```python
from build123d import *

# Parameters (mm, degrees)
SKETCH4_R           = 63.754
BOSS_EXTRUDE1_DEPTH = 62.5856
SKETCH5_R           = 34.671
BOSS_EXTRUDE2_DEPTH = 58.42


with BuildPart() as part:
    # Sketch1 → Revolve1 (revolve)
    with BuildSketch(Plane.XY):
        Polygon((-83.185, -63.754), (-31.2928, -63.754), (-31.2928, -57.0357), (-83.185, -57.3786), align=None)
        Polygon((83.185, -57.3786), (31.2928, -57.0357), (31.2928, -63.754), (83.185, -63.754), align=None)
    revolve(axis=Axis((-83.185, 0, 0), (1, 0, 0)))



with BuildPart() as body_2:
    # Sketch2 → Revolve2 (revolve)
    with BuildSketch(Plane.XY):
        Polygon((30.3149, 93.98), (30.0863, 58.42), (34.671, 58.42), (34.671, 93.98), align=None)
    revolve(axis=Axis((0, 0, 0), (0, 1, 0)))


with BuildPart() as part_1:
    add(part.part)

    add(body_2.part)  # Boss-Extrude1 merges body 2
    # Sketch4 → Boss-Extrude1 (add)
    with BuildSketch(Plane(origin=(-31.2928, 0, 0), x_dir=(0, 0, -1), z_dir=(1, 0, 0))):
        Circle(SKETCH4_R)
    extrude(amount=BOSS_EXTRUDE1_DEPTH)

    # Sketch5 → Boss-Extrude2 (add)
    with BuildSketch(Plane.XZ.offset(-58.42)):
        Circle(SKETCH5_R)
    extrude(amount=BOSS_EXTRUDE2_DEPTH)

    # Sketch6 → Cut-Revolve1 (revolve, cut)
    with BuildSketch(Plane.XY):
        Polygon((-83.185, -57.3786), (-31.2928, -57.0357), (-31.2928, -51.1302), (31.2928, -51.1302), (31.2928, -57.0357), (83.185, -57.3786), (83.185, 0), (-83.185, 0), align=None)
    revolve(axis=Axis((83.185, 0, 0), (-1, 0, 0)), mode=Mode.SUBTRACT)

    # Sketch7 → Cut-Revolve2 (revolve, cut)
    with BuildSketch(Plane.XY):
        Polygon((30.3149, 93.98), (30.0863, 58.42), (26.2509, 58.42), (26.2509, 0), (0, 0), (0, 93.98), align=None)
    revolve(axis=Axis((0, 0, 0), (0, 1, 0)), mode=Mode.SUBTRACT)


solid = part_1.part
```
For this review, take the finished solid that the model builds, in its own axes (mm). Round coordinates to 2 decimals unless told otherwise and drop trailing zeros. Write each loop counter-clockwise with the first axis right and the second up, starting at its lowest first coordinate (ties: lowest second). Pieces come first, ordered by that corner, then holes.
1) For line 1 along Z through (x, y) = (-17, 0); line 2 along Y through (x, z) = (7.5, 0); line 3 along X through (y, z) = (-13.5, 52.5), list the stretches that pass through material, from the lowest coordinate up.
Answer below:
line 1: z = -63.75 to -51.13, 51.13 to 63.75
line 2: y = -63.75 to -51.13
line 3: x = -31.29 to 31.29
2) Take a section at A-A on x = 54. Give the boundary of the cut face in (y, z), then the cut area to 3 significant figures.
Answer below:
outline: circle Ø127.51 at (0, 0); hole circle Ø114.37 at (0, 0)
area: 2,500 mm2
3) Mouldability with a two-part tool opening along Z and no side actions: class faces 1 (the face through (25.039, 52.662, -7.885)), 2 (the face through (83.185, 57, -10)), 3 (the face through (-27.51, 74.02, -21.1)) as +Z half, -Z half, draft (parallel to the pull), parting line (faces both ways), or undercut.
Answer below:
face 1: undercut
face 2: draft
face 3: parting line
4) Insertion check: pin 1 Ø6 at (y, z) = (40, -35) entering from -X; pin 2 Ø2 at (x, y) = (-65.5, -46.5) entering from -Z; pin 3 Ø19 at (x, z) = (-14.5, 2) entering from +Y. Each pin has a flat end and moves straight along its axis. Give the tip position at first contact, or say it passes through.
Answer below:
pin 1: stops at x = -31.29
pin 2: stops at z = -44.66
pin 3: stops at y = -49.82
